from build123d import *

# Parameters (mm, degrees)
CYLINDER002_R     = 2
CYLINDER002_DEPTH = 10
BOX_W             = 6
BOX_H             = 3
BOX_DEPTH         = 10
CYLINDER_R        = 8.5
CYLINDER_DEPTH    = 11
POCKET_DEPTH      = 6


with BuildPart() as cilindro002:
    # Cylinder002 → Cylinder002 (new body)
    with BuildSketch(Plane(origin=(0, 10.2, 8.25), x_dir=(1, 0, 0), z_dir=(0, -1, 0))):
        Circle(CYLINDER002_R)
    extrude(amount=CYLINDER002_DEPTH)


with BuildPart() as cubo:
    # Box → Box (new body)
    with BuildSketch(Plane(origin=(-3, 3, 2.5), x_dir=(1, 0, 0), z_dir=(0, 0, 1))):
        with Locations((3, 1.5)):
            Rectangle(BOX_W, BOX_H)
    extrude(amount=BOX_DEPTH)


with BuildPart() as body:
    # Cylinder → Cylinder (new body)
    with BuildSketch(Plane.XY):
        Circle(CYLINDER_R)
    extrude(amount=CYLINDER_DEPTH)

    # Cut: cut Cubo
    add(cubo.part, mode=Mode.SUBTRACT)

    # Cut002: cut Cilindro002
    add(cilindro002.part, mode=Mode.SUBTRACT)


with BuildPart() as body_1:
    # Cut002 placement: moved
    add(body.part.moved(Location((0, 0, -1))))


with BuildPart() as body_2:
    # BaseFeature placement: moved
    add(body_1.part.moved(Location((0, 0, 1))))

    # Sketch → Pocket (cut)
    with BuildSketch(Plane.XY.offset(11)):
        with BuildLine():
            ThreePointArc((-1.813836, 2), (-2.7, 0), (-1.813836, -2))
            Line((1.813836, -2), (-1.813836, -2))
            ThreePointArc((1.813836, -2), (2.7, 0), (1.813836, 2))
            Line((-1.813836, 2), (1.813836, 2))
        make_face()
    extrude(amount=-POCKET_DEPTH, mode=Mode.SUBTRACT)


solid = body_2.part
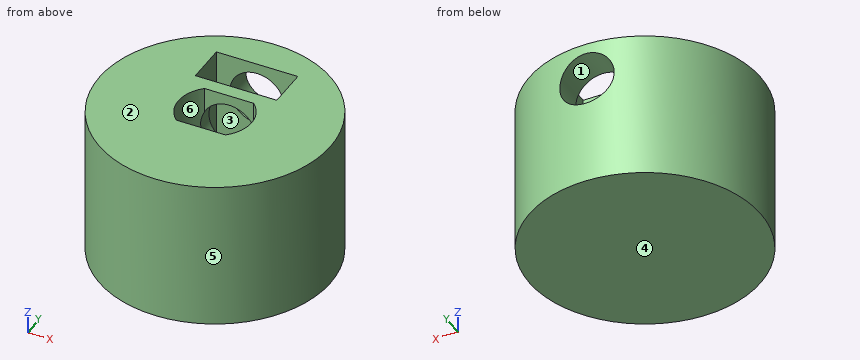
Verification items for the finished model (mm, model axes). Face numbers are marked on the shaded views. A direction names the side the tool comes from. Give positions to 0.01 mm unless a question says otherwise; leave off trailing zeros. Order: outer loops, then holes, each group sorted by start corner. A loop starts at its lowest first (then second) coordinate and runs counter-clockwise, first axis right, second up. Notation, with made-up numbers: M 89,-12 L 113,-12 A33 ccw 113,20 Z; hole C -36,57.25 d2. An arc over 180 degrees is marked long. Use one line per item in the form item = value. Start each with the question number.
Q1. Access from +Z, -Z, +X, -X, +Y, -Y to the whole of each face (thin tool, end or side, straight path). Record for the marked faces 1, 2 and 3.
Q2. Section check C-C (y = 0). Enter the section's corners in (x, z).
Q3. Scan lines: line 1 along Z through (x, y) = (0, 6.7); line 2 along Y through (x, z) = (0, 7.75); line 3 along X through (y, z) = (7.1, 8.25). Record each from-to range of solid material in increasing order. Write a range as [from, to].
Q4. Section check B-B (z = 6). Enter the section's corners in (x, y), then the cut area to 3 significant figures.
Q5. Section check D-D (z = 8.25). Enter the section's corners in (x, y).
Q6. Section check A-A (x = 0). Enter the section's corners in (y, z).
Q7. Go/stop test with flat-tipped pins: pin 1 Ø4 at (x, z) = (-6, 3.5) entering from -Y; pin 2 Ø0.9 at (y, z) = (5, 8) entering from -X; pin 3 Ø3.5 at (y, z) = (4.5, 6) entering from +X. Record where each tip stops, or that it passes through.
Q8. Mould release check, pull along Y, two halves, no side actions. Record for the marked faces 4, 5 and 6: +Y half, -Y half, draft (parallel to the pull), parting line (faces both ways), or undercut.
Evaluation:
q1.face_1 = +Y
q1.face_2 = +Z, +X, -X, +Y, -Y
q1.face_3 = +Z
q2.outline = M -8.5,0 L 8.5,0 L 8.5,11 L 2.7,11 L 2.7,5 L -2.7,5 L -2.7,11 L -8.5,11 Z
q3.line_1 = [0, 6.25], [10.25, 11]
q3.line_2 = [-8.5, -2]
q3.line_3 = [-4.67, -2], [2, 4.67]
q4.outline = C 0,0 d17; hole M -3,3 L 3,3 L 3,6 L -3,6 Z; hole M -1.81,-2 L 1.81,-2 A2.7 ccw 1.81,2 L -1.81,2 A2.7 ccw Z
q4.area = 190 mm2
q5.outline = M -3,3 L -3,6 L -2,6 L -2,8.26 A8.5 ccw long 2,8.26 L 2,6 L 3,6 L 3,3 L 2,3 L 2,1.81 A2.7 cw 1.81,-2 L -1.81,-2 A2.7 cw -2,1.81 L -2,3 Z
q6.outline = M -8.5,0 L 8.5,0 L 8.5,6.25 L 6,6.25 L 6,2.5 L 3,2.5 L 3,6.25 L 2,6.25 L 2,5 L -2,5 L -2,11 L -8.5,11 Z; M 2,10.25 L 3,10.25 L 3,11 L 2,11 Z; M 6,10.25 L 8.5,10.25 L 8.5,11 L 6,11 Z
q7.pin_1 = -7.5
q7.pin_2 = -7.18
q7.pin_3 = 8.04
q8.face_4 = draft
q8.face_5 = parting line
q8.face_6 = undercut
